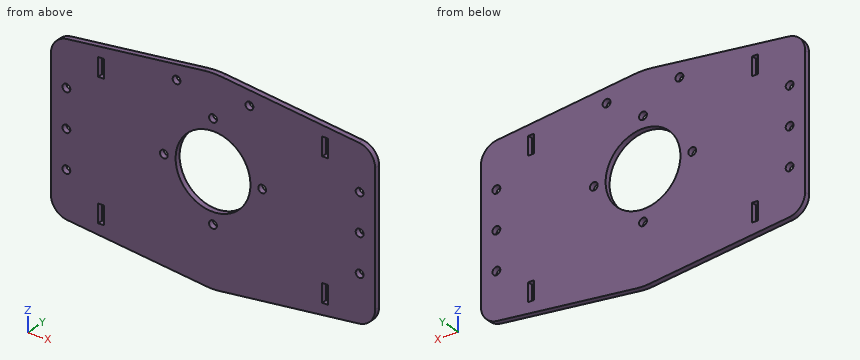
from build123d import *

# Parameters (mm, degrees)
SKETCH1_R                = 20.55
SKETCH1_R_2              = 1
SKETCH1_W                = 3.1
SKETCH1_H                = 10.1
BASE_FLANGE1_DEPTH       = 3
FILLET1_R                = 10
M4_CLEARANCE_HOLE2_D     = 4.3
M4_CLEARANCE_HOLE2_DEPTH = 136
M4_CLEARANCE_HOLE2_TIP   = 1.291850331


# Sheet-metal steps are written as plain solids
with BuildPart() as part:
    # Sketch1 → Base-Flange1 (new body)
    with BuildSketch(Plane(origin=(0, 0, 0), x_dir=(1, 0, 0), z_dir=(0, 1, 0))):
        with BuildLine():
            Line((-89, -40), (-89, 50))
            Line((-89, 50), (-3.349708355, 59.623628275))
            ThreePointArc((-3.349708355, 59.623628275), (0, 59.811223911), (3.349708355, 59.623628275))
            Line((3.349708355, 59.623628275), (89, 50))
            Line((89, 50), (89, -40))
            Line((89, -40), (5.17352088, -49.701618334))
            ThreePointArc((5.17352088, -49.701618334), (0, -50), (-5.17352088, -49.701618334))
            Line((-5.17352088, -49.701618334), (-89, -40))
        make_face()
        with Locations(Location((0, 0, 0), (0, 0, 270))):
            Circle(SKETCH1_R, mode=Mode.SUBTRACT)
        with Locations(Location((0, 27, 0), (0, 0, 270))):
            Circle(SKETCH1_R_2, mode=Mode.SUBTRACT)
        with Locations(Location((-80.5, 25.5, 0), (0, 0, 270))):
            Circle(SKETCH1_R_2, mode=Mode.SUBTRACT)
        with Locations(Location((-80.5, 4.75, 0), (0, 0, 270))):
            Circle(SKETCH1_R_2, mode=Mode.SUBTRACT)
        with Locations(Location((-80.5, -16, 0), (0, 0, 270))):
            Circle(SKETCH1_R_2, mode=Mode.SUBTRACT)
        with Locations(Location((80.5, -16, 0), (0, 0, 90))):
            Circle(SKETCH1_R_2, mode=Mode.SUBTRACT)
        with Locations(Location((80.5, 4.75, 0), (0, 0, 90))):
            Circle(SKETCH1_R_2, mode=Mode.SUBTRACT)
        with Locations(Location((80.5, 25.5, 0), (0, 0, 90))):
            Circle(SKETCH1_R_2, mode=Mode.SUBTRACT)
        with Locations(Location((27, 0, 0), (0, 0, 270))):
            Circle(SKETCH1_R_2, mode=Mode.SUBTRACT)
        with Locations(Location((0, -27, 0), (0, 0, 270))):
            Circle(SKETCH1_R_2, mode=Mode.SUBTRACT)
        with Locations(Location((-27, 0, 0), (0, 0, 270))):
            Circle(SKETCH1_R_2, mode=Mode.SUBTRACT)
        with Locations(Location((20, -40, 0), (0, 0, 270))):
            Circle(SKETCH1_R_2, mode=Mode.SUBTRACT)
        with Locations(Location((-20, -40, 0), (0, 0, 270))):
            Circle(SKETCH1_R_2, mode=Mode.SUBTRACT)
        with Locations((-61.5, 42)):
            Rectangle(SKETCH1_W, SKETCH1_H, mode=Mode.SUBTRACT)
        with Locations((-61.5, -32.5)):
            Rectangle(SKETCH1_W, SKETCH1_H, mode=Mode.SUBTRACT)
        with Locations((61.5, -32.5)):
            Rectangle(SKETCH1_W, SKETCH1_H, mode=Mode.SUBTRACT)
        with Locations((61.5, 42)):
            Rectangle(SKETCH1_W, SKETCH1_H, mode=Mode.SUBTRACT)
    extrude(amount=-BASE_FLANGE1_DEPTH)

    # Fillet1
    fillet1_edges = [part.edges().sort_by_distance(p)[0] for p in [
        (89, -1.5, -50),
        (89, -1.5, 40),
        (-89, -1.5, 40),
        (-89, -1.5, -50),
    ]]
    fillet(fillet1_edges, radius=FILLET1_R)

    # M4 Clearance Hole2
    with Locations(Plane(origin=(0, 0, 0), x_dir=(1, 0, 0), z_dir=(0, 1, 0))):
        with Locations((-27, 0), (0, 27), (27, 0), (0, -27), (20, -40), (-20, -40), (80.5, -16), (80.5, 25.5), (80.5, 4.75), (-80.5, 25.5), (-80.5, 4.75), (-80.5, -16)):
            Hole(M4_CLEARANCE_HOLE2_D / 2, depth=M4_CLEARANCE_HOLE2_DEPTH)
            with Locations((0, 0, -(M4_CLEARANCE_HOLE2_DEPTH + M4_CLEARANCE_HOLE2_TIP / 2))):  # 118° drill point
                Cone(0, M4_CLEARANCE_HOLE2_D / 2, M4_CLEARANCE_HOLE2_TIP, mode=Mode.SUBTRACT)


solid = part.part
Could you check a few things on this model? Use its own coordinates, in mm. Round coordinates to 2 decimals unless told otherwise and drop trailing zeros. Order: outer loops, then holes, each group sorted by start corner. A loop starts at its lowest first (then second) coordinate and runs counter-clockwise, first axis right, second up.
Q1. Please list where these lines run through material, in increasing order: probe 1 along X at (y, z) = (-2.35, -39); probe 2 along X at (y, z) = (-1.8, -5.5); probe 3 along X at (y, z) = (-0.65, -43).
Geometry says:
probe 1: x = -89 to -63.05, -59.95 to 59.95, 63.05 to 89
probe 2: x = -89 to -82.51, -78.49 to -19.8, 19.8 to 78.49, 82.51 to 89
probe 3: x = -88.81 to -63.05, -59.95 to 59.95, 63.05 to 88.81
Q2. Imagine slicing it at C-C, the plane x = 27. List the corners of the cut face in (y, z) for me, then the cut area to 3 significant figures.
Geometry says:
outline: (-3, -56.97) - (0, -56.97) - (0, -2.15) - (-3, -2.15) - close; (-3, 2.15) - (0, 2.15) - (0, 47.18) - (-3, 47.18) - close
area: 300 mm2
Q3. Imagine slicing it at A-A, the plane z = 0. List the corners of the cut face in (x, y) for me, then the cut area to 3 significant figures.
Geometry says:
outline: (-89, -3) - (-29.15, -3) - (-29.15, 0) - (-89, 0) - close; (-24.85, -3) - (-20.55, -3) - (-20.55, 0) - (-24.85, 0) - close; (20.55, -3) - (24.85, -3) - (24.85, 0) - (20.55, 0) - close; (29.15, -3) - (89, -3) - (89, 0) - (29.15, 0) - close
area: 385 mm2
Q4. I'm going to push a flat-ended pin straight in: P1, Ø3.5, axis at x = -20, z = 40, coming from the +Y side. Where does the tip first touch, or does it pass through?
Geometry says:
P1: passes through
Q5. Imagine slicing it at B-B, the plane x = 0. List the corners of the cut face in (y, z) for me, then the cut area to 3 significant figures.
Geometry says:
outline: (-3, -59.81) - (0, -59.81) - (0, -29.15) - (-3, -29.15) - close; (-3, -24.85) - (0, -24.85) - (0, -20.55) - (-3, -20.55) - close; (-3, 20.55) - (0, 20.55) - (0, 24.85) - (-3, 24.85) - close; (-3, 29.15) - (0, 29.15) - (0, 50) - (-3, 50) - close
area: 180 mm2
Q6. Imagine slicing it at D-D, the plane z = -14. List the corners of the cut face in (x, y) for me.
Geometry says:
outline: (-89, -3) - (-15.04, -3) - (-15.04, 0) - (-89, 0) - close; (15.04, -3) - (89, -3) - (89, 0) - (15.04, 0) - close
